CAD build for the part. Positions are in the model's coordinates, mm. A direction names the side the tool comes from. Round coordinates to 2 decimals unless told otherwise and drop trailing zeros. Order: outer loops, then holes, each group sorted by start corner. A loop starts at its lowest first (then second) coordinate and runs counter-clockwise, first axis right, second up. Notation, with made-up numbers: (56.5, 49) -> (105.5, 49) arc R32 ccw to (105.5, 87) -> close; hole circle Ø5 at (-34.75, 39). An arc over 180 degrees is marked (long way). Answer as CSV lines item,"result". Start each with the question number.
from build123d import *

# Parameters (mm, degrees)
F0_R     = 9.525
F1_DEPTH = 9.525
F2_R     = 1.905
F3_DEPTH = 25.4


with BuildPart() as f1:
    # F0 (on Top) → F1 (new body)
    with BuildSketch(Plane.XY):
        with BuildLine():
            Line((-28.575, -12.7), (-28.575, -19.05))
            Line((-28.575, -19.05), (0, -19.05))
            Line((0, -19.05), (28.575, -19.05))
            Line((28.575, -19.05), (28.575, -12.7))
            Line((28.575, -12.7), (19.05, -12.7))
            ThreePointArc((19.05, -12.7), (14.559872, -10.840128), (12.7, -6.35))
            Line((12.7, -6.35), (12.7, 12.7))
            ThreePointArc((12.7, 12.7), (8.980256, 21.680256), (0, 25.4))
            ThreePointArc((0, 25.4), (-8.980256, 21.680256), (-12.7, 12.7))
            Line((-12.7, 12.7), (-12.7, -6.35))
            ThreePointArc((-12.7, -6.35), (-14.559872, -10.840128), (-19.05, -12.7))
            Line((-19.05, -12.7), (-28.575, -12.7))
        make_face()
        with Locations((0, 12.7)):
            Circle(F0_R, mode=Mode.SUBTRACT)
    extrude(amount=F1_DEPTH)

    # F2 (on face) → F3 (cut)
    with BuildSketch(Plane.XZ.offset(19.05)):
        with Locations((-23.8125, 4.7625)):
            Circle(F2_R)
        with Locations((23.8125, 4.7625)):
            Circle(F2_R)
    extrude(amount=-F3_DEPTH, mode=Mode.SUBTRACT)


solid = f1.part
Item 1: Band-saw the part on B-B, the plane y = 19. Give the cut face in (x, z) (3 decimals).
Item 2: Band-saw the part on D-D, the plane z = 8.5. Give the cut face in (x, y) (3 decimals), and give its area (3 significant figures).
Item 3: Band-saw the part on A-A, the plane z = 4. Give the cut face in (x, y) (3 decimals), and give its area (3 significant figures).
Item 4: Tool access for faces 1 (the flat face through (26, -12.7, 5)), 2 (the flat face through (-24, -12.7, 7)), 3 (the cylindrical face through (25.57, -15.92, 4.03)): list every direction of +Z, -Z, +X, -X, +Y, -Y with a clear straight run to the whole face (end or side of a thin tool).
Item 5: Band-saw the part on C-C, the plane x = -22.5. Give the cut face in (y, z) (3 decimals), and give its area (3 significant figures).
Item 6: Mould opens along X. For faces 4 (the cylindrical face through (-2.06, 3.4, 4.7)), 5 (the flat face through (0, -6, 0)), 6 (the cylindrical face through (-14.51, -10.79, 4.7)) say: released by +X, released by -X, zero draft, split by the parting line, or undercut.
Item 7: Pin check, flat tips, straight feed: pin 1 (1.5 mm diameter, centred on y = 19, z = 1, fed in from +X); pin 2 (2 mm diameter, centred on y = -12.5, z = 5, fed in from +X) (3 decimals); pin 3 (3 mm diameter, centred on x = -26, z = 4, fed in from +Y); pin 4 (3 mm diameter, centred on y = 4.5, z = 6, fed in from +X). Stop position of each tip, or through.
Item 8: Probe line 1 (Y direction, x = 0, z = 4.25) (3 decimals); line 2 (X direction, y = 1.5, z = 2.75); line 3 (X direction, y = 18.5, z = 8.25). List the from-to ranges inside material, lowest first.
Values:
1,outline,"(-11.027, 0) -> (-7.144, 0) -> (-7.144, 9.525) -> (-11.027, 9.525) -> close; (7.144, 0) -> (11.027, 0) -> (11.027, 9.525) -> (7.144, 9.525) -> close"
2,outline,"(-28.575, -19.05) -> (28.575, -19.05) -> (28.575, -12.7) -> (19.05, -12.7) arc R6.35 cw to (12.7, -6.35) -> (12.7, 12.7) arc R12.7 ccw to (-12.7, 12.7) -> (-12.7, -6.35) arc R6.35 cw to (-19.05, -12.7) -> (-28.575, -12.7) -> close; hole circle Ø19.05 at (0, 12.7)"
2,area,"994 mm²"
3,outline,"(-28.575, -19.05) -> (-25.558, -19.05) -> (-25.558, -12.7) -> (-28.575, -12.7) -> close; (-22.067, -19.05) -> (22.067, -19.05) -> (22.067, -12.7) -> (19.05, -12.7) arc R6.35 cw to (12.7, -6.35) -> (12.7, 12.7) arc R12.7 ccw to (-12.7, 12.7) -> (-12.7, -6.35) arc R6.35 cw to (-19.05, -12.7) -> (-22.067, -12.7) -> close; (25.558, -19.05) -> (28.575, -19.05) -> (28.575, -12.7) -> (25.558, -12.7) -> close; hole circle Ø19.05 at (0, 12.7)"
3,area,"949 mm²"
4,face 1,"+Z, -Z, +X, +Y"
4,face 2,"+Z, -Z, -X, +Y"
4,face 3,"+Y, -Y"
5,outline,"(-19.05, 0) -> (-12.7, 0) -> (-12.7, 3.382) -> (-19.05, 3.382) -> close; (-19.05, 6.143) -> (-12.7, 6.143) -> (-12.7, 9.525) -> (-19.05, 9.525) -> close"
5,area,"42.9 mm²"
6,face 4,"undercut"
6,face 5,"zero draft"
6,face 6,"released by -X"
7,pin 1,"x = 11.42"
7,pin 2,"x = 28.575"
7,pin 3,"y = -12.7"
7,pin 4,"x = 12.7"
8,line 1,"-19.05 to 3.175, 22.225 to 25.4"
8,line 2,"-12.7 to 12.7"
8,line 3,"-11.3 to -7.56, 7.56 to 11.3"
